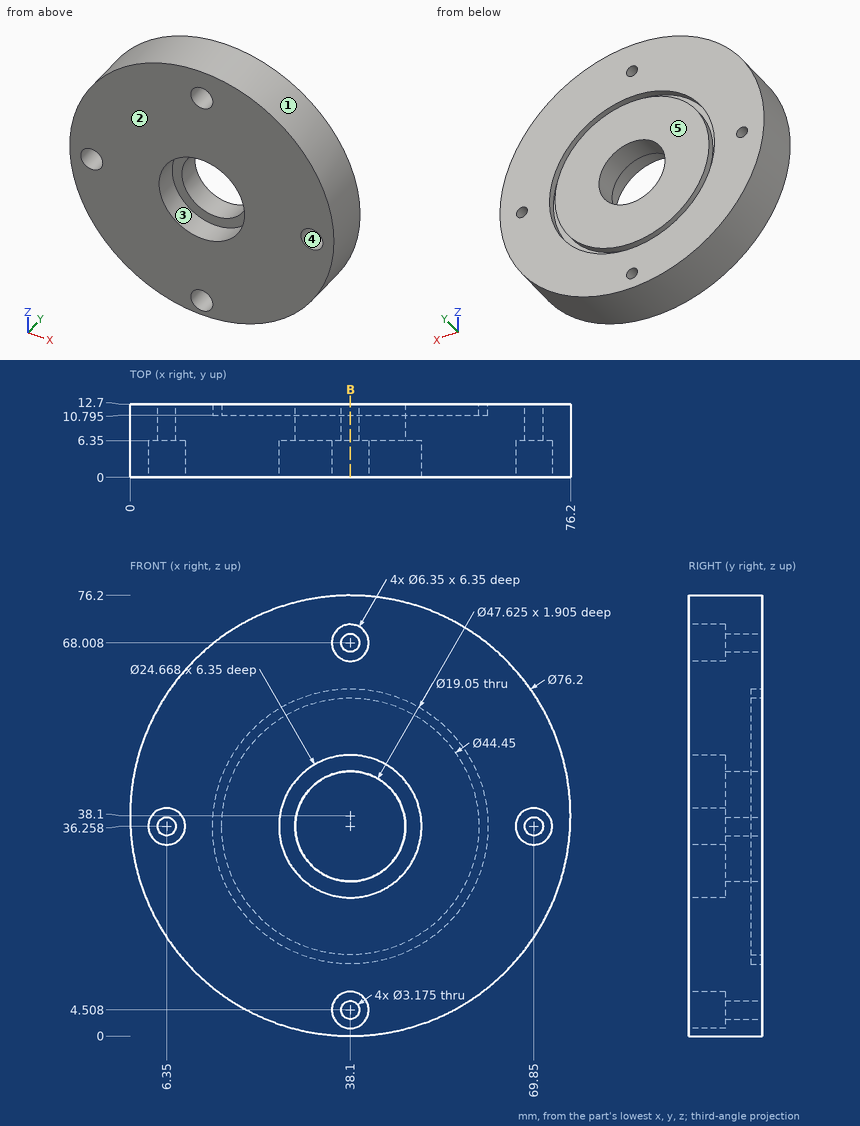
Verification items for this drawing (mm, ordinates from the low corner). A direction names the side the tool comes from. Round coordinates to 2 decimals unless told otherwise and drop trailing zeros.
1) Tool access check on the marked faces 4 and 5. Record the directions out of +Z, -Z, +X, -X, +Y, -Y that give a thin tool (end or side, any length) a straight path to the whole face; none if there is none.
Geometry says:
face 4: -Y
face 5: +Z, -Z, +X, -X, +Y
2) Depth check by flat-ended pin: pin 1 (3 mm diameter, centred on x = 38.5, z = 3.5, fed in from -Y); pin 2 (1 mm diameter, centred on x = 67, y = 11, fed in from +Z); pin 3 (6 mm diameter, centred on x = 16.5, y = 1.5, fed in from +Z). Enter the tip coordinate at first touch or a pass-through.
Geometry says:
pin 1: stops at y = 6.35
pin 2: stops at z = 63.5
pin 3: stops at z = 71.35
3) Draft check along Z on the marked faces 1, 2 and 3. Enter one of: +Z half, -Z half, draft (parallel to the pull), parting line (faces both ways), or undercut.
Geometry says:
face 1: parting line
face 2: draft
face 3: undercut
4) Cross-section at B-B, the plane x = 38.1. Give the number of separate pieces and of enclosed holes in the cut face, plus the area to 3 significant figures.
Geometry says:
separate pieces: 4
enclosed holes: 0
area: 563 mm2
5) Material ranges on line 1 (Z direction, x = 38.1, y = 4.75) (1 decimal); line 2 (X direction, y = 12, z = 32); line 3 (Z direction, x = 33, y = 11) (1 decimal), recorded low to high.
Geometry says:
line 1: z = 0 to 1.3, 7.7 to 23.9, 48.6 to 64.8, 71.2 to 76.2
line 2: x = 0.49 to 14.67, 16.29 to 29.58, 46.62 to 59.91, 61.53 to 75.71
line 3: z = 0.3 to 13, 14.6 to 28.2, 44.3 to 57.9, 59.5 to 75.9
